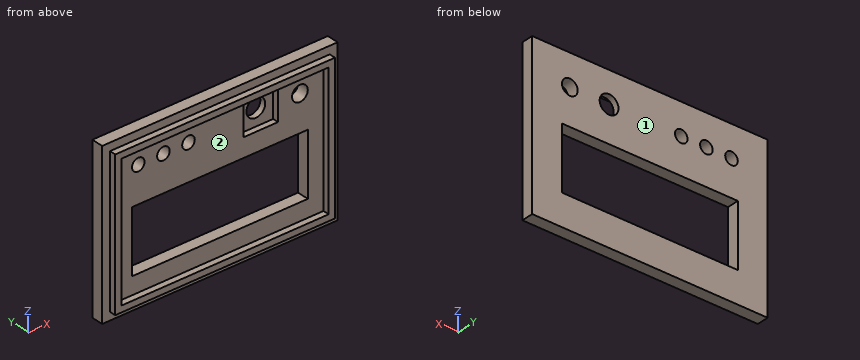
```python
from build123d import *

# Parameters (mm, degrees)
SKETCH1_W               = 95.25
SKETCH1_H               = 65.405
SKETCH1_R               = 2.54
SKETCH1_R_2             = 3.175
SKETCH1_R_3             = 3.81
SKETCH1_W_2             = 71.12
SKETCH1_H_2             = 25.4
BOSS_EXTRUDE1_DEPTH     = 4.7625
SKETCH3_W               = 88.9
SKETCH3_H               = 59.055
SKETCH3_W_2             = 83.82
SKETCH3_H_2             = 53.975
BOSS_EXTRUDE2_DEPTH     = 2.54
CUT_EXTRUDE1_DEPTH      = 116.641938462
CUT_EXTRUDE1_DEPTH_BACK = 2.38125
SKETCH2_W               = 13.97
SKETCH2_H               = 13.97


with BuildPart() as part:
    # Sketch1 → Boss-Extrude1 (new body)
    with BuildSketch(Plane(origin=(0, 0, 0), x_dir=(1, 0, 0), z_dir=(0, 1, 0))):
        with Locations((47.625, 32.7025)):
            Rectangle(SKETCH1_W, SKETCH1_H)
        with Locations(Location((34.925, 12.7, 0), (0, 0, 90))):
            Circle(SKETCH1_R, mode=Mode.SUBTRACT)
        with Locations(Location((14.605, 12.7, 0), (0, 0, 90))):
            Circle(SKETCH1_R, mode=Mode.SUBTRACT)
        with Locations(Location((24.765, 12.7, 0), (0, 0, 90))):
            Circle(SKETCH1_R, mode=Mode.SUBTRACT)
        with Locations(Location((80.01, 12.7, 0), (0, 0, 90))):
            Circle(SKETCH1_R_2, mode=Mode.SUBTRACT)
        with Locations(Location((64.135, 12.7, 0), (0, 0, 90))):
            Circle(SKETCH1_R_3, mode=Mode.SUBTRACT)
        with Locations((47.625, 40.005)):
            Rectangle(SKETCH1_W_2, SKETCH1_H_2, mode=Mode.SUBTRACT)
    extrude(amount=BOSS_EXTRUDE1_DEPTH)

    # Sketch3 → Boss-Extrude2 (add)
    with BuildSketch(Plane.XZ):
        with Locations((47.625, -32.7025)):
            Rectangle(SKETCH3_W, SKETCH3_H)
        with Locations((47.625, -32.7025)):
            Rectangle(SKETCH3_W_2, SKETCH3_H_2, mode=Mode.SUBTRACT)
    extrude(amount=BOSS_EXTRUDE2_DEPTH)

    # Sketch2 → Cut-Extrude1 (cut, two sides: drawn at the far end of the back side and taken through both)
    with BuildSketch(Plane.XZ.offset(-CUT_EXTRUDE1_DEPTH_BACK)):
        with Locations((64.135, -12.7)):
            Rectangle(SKETCH2_W, SKETCH2_H)
    extrude(amount=CUT_EXTRUDE1_DEPTH + CUT_EXTRUDE1_DEPTH_BACK, mode=Mode.SUBTRACT)


solid = part.part
```
Part model, mm, in its own coordinate system. Face numbers are marked on the shaded views. Round coordinates to 2 decimals unless told otherwise and drop trailing zeros. Loops run counter-clockwise (first coordinate to the right, second up) from the corner with the lowest first, then second, coordinate; pieces in that order, holes last. Notation, with made-up numbers: (-20, 29) -> (37, 29) arc R25 cw to (37, 46) -> close; hole circle Ø6 at (18.5, 27). An arc over 180 degrees is marked (long way). Use a Markdown table: item, result.
1) Drop flat-ended pins along their axis: pin 1 Ø6.5 at (x, z) = (24.765, -12.7) entering from +Y; pin 2 Ø5.5 at (x, z) = (80.01, -12.7) entering from +Y; pin 3 Ø8 at (x, z) = (34.925, -12.7) entering from -Y; pin 4 Ø3 at (y, z) = (-2, -32) entering from +X (3 decimals). Give the stop position or say it passes through.
The answers:
| item | result |
|---|---|
| pin 1 | stops at y = 4.76 |
| pin 2 | passes through |
| pin 3 | stops at y = 0 |
| pin 4 | stops at x = 92.075 |
2) Cut at D-D, the plane z = -12.7. State how many separate pieces and enclosed holes the cut face has, and give its area (3 significant figures).
The answers:
| item | result |
|---|---|
| separate pieces | 6 |
| enclosed holes | 0 |
| area | 312 mm2 |
3) Pull direction Z, two halves, no side cores. Call the marked faces 1 and 2: pulls with the +Z half, pulls with the -Z half, needs draft (parallel to the pull), parting line crosses it, or undercut.
The answers:
| item | result |
|---|---|
| face 1 | needs draft |
| face 2 | undercut |
4) Probe line 1 (X direction, y = 1.6, z = -12.7) (3 decimals); line 2 (X direction, y = 2.7, z = -12.7) (3 decimals); line 3 (Z direction, x = 80.01, y = 3.2) (3 decimals). List the from-to ranges inside material, lowest first. Write a range as [from, to].
The answers:
| item | result |
|---|---|
| line 1 | x = [0, 12.065], [17.145, 22.225], [27.305, 32.385], [37.465, 57.15], [71.12, 76.835], [83.185, 95.25] |
| line 2 | x = [0, 12.065], [17.145, 22.225], [27.305, 32.385], [37.465, 60.325], [67.945, 76.835], [83.185, 95.25] |
| line 3 | z = [-65.405, -52.705], [-27.305, -15.875], [-9.525, 0] |
5) Cut at C-C, the plane x = 46. List the corners of the cut face in (y, z) (1 decimal).
The answers:
| item | result |
|---|---|
| outline | (-2.5, -62.2) -> (0, -62.2) -> (0, -65.4) -> (4.8, -65.4) -> (4.8, -52.7) -> (0, -52.7) -> (0, -59.7) -> (-2.5, -59.7) -> close; (-2.5, -5.7) -> (0, -5.7) -> (0, -27.3) -> (4.8, -27.3) -> (4.8, 0) -> (0, 0) -> (0, -3.2) -> (-2.5, -3.2) -> close |
6) Cut at A-A, the plane x = 80.01. List the corners of the cut face in (y, z) (1 decimal).
The answers:
| item | result |
|---|---|
| outline | (-2.5, -62.2) -> (0, -62.2) -> (0, -65.4) -> (4.8, -65.4) -> (4.8, -52.7) -> (0, -52.7) -> (0, -59.7) -> (-2.5, -59.7) -> close; (-2.5, -5.7) -> (0, -5.7) -> (0, -9.5) -> (4.8, -9.5) -> (4.8, 0) -> (0, 0) -> (0, -3.2) -> (-2.5, -3.2) -> close; (0, -27.3) -> (4.8, -27.3) -> (4.8, -15.9) -> (0, -15.9) -> close |
